Input: part model. Units: mm. Frame: model coordinates. Face numbers are marked on the shaded views. A direction names the side the tool comes from. Coordinates: 2 decimals unless noted, no trailing zeros. Write each loop counter-clockwise with the first axis right and the second up, starting at its lowest first coordinate (ties: lowest second). Pieces come first, ordered by that corner, then holes. Notation, with made-up numbers: (30, -36) - (71, -36) arc R23 ccw to (71, -11) - close; hole circle Ø4 at (14, 64.25). An arc over 180 degrees is marked (long way). Use CSV: the item, a comma, the result in double quotes.
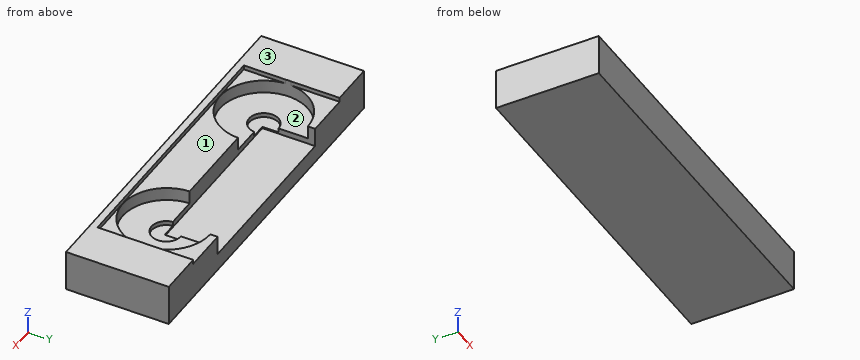
```python
from build123d import *

# Parameters (mm, degrees)
F0_W      = 304.8
F0_H      = 88.9
F1_DEPTH  = 35.56
F2_R      = 38.1
F3_DEPTH  = 15.24
F4_R      = 38.1
F5_DEPTH  = 15.24
F6_W      = 152.4
F6_H      = 20.32
F7_DEPTH  = 45.72
F8_W      = 228.6
F8_H      = 82.7938915014
F9_DEPTH  = 3.81
F10_R     = 12.7
F11_DEPTH = 3.81
F12_R     = 12.7
F13_DEPTH = 3.81


# Not quite as in the source:
# - a feature of the source that left no trace in its solid (it failed there, or was rolled back) is left out


with BuildPart() as f1:
    # F0 (on Top) → F1 (new body)
    with BuildSketch(Plane.XY):
        Rectangle(F0_W, F0_H)
    extrude(amount=F1_DEPTH)

    # F2 (on face) → F3 (cut)
    with BuildSketch(Plane.XY.offset(35.56)):
        with Locations((75.4419565201, 0)):
            Circle(F2_R)
    extrude(amount=-F3_DEPTH, mode=Mode.SUBTRACT)

    # F4 (on face) → F5 (cut)
    with BuildSketch(Plane.XY.offset(35.56)):
        with Locations((-76.2725099921, 0)):
            Circle(F4_R)
    extrude(amount=-F5_DEPTH, mode=Mode.SUBTRACT)

    # F6 (on face) → F7 (cut)
    with BuildSketch(Plane(origin=(0, 44.45, 0), x_dir=(-1, 0, 0), z_dir=(0, 1, 0))):
        with Locations((0, 25.4)):
            Rectangle(F6_W, F6_H)
    extrude(amount=-F7_DEPTH, mode=Mode.SUBTRACT)

    # F8 (on face) → F9 (cut)
    with BuildSketch(Plane.XY.offset(35.56)):
        with Locations((0, 3.0530542493)):
            Rectangle(F8_W, F8_H)
    extrude(amount=-F9_DEPTH, mode=Mode.SUBTRACT)

    # F10 (on face) → F11 (cut)
    with BuildSketch(Plane.XY.offset(20.32)):
        with Locations((-76.2, 0)):
            Circle(F10_R)
    extrude(amount=-F11_DEPTH, mode=Mode.SUBTRACT)

    # F12 (on face) → F13 (cut)
    with BuildSketch(Plane.XY.offset(20.32)):
        with Locations((76.2, 0)):
            Circle(F12_R)
    extrude(amount=-F13_DEPTH, mode=Mode.SUBTRACT)


solid = f1.part
```
(1) Pin query (flat end, axial travel): pin 1 Ø23 at (x, y) = (-76.2, 0) entering from -Z; pin 2 Ø10 at (x, y) = (-24.5, 2) entering from +Z; pin 3 Ø8.5 at (x, z) = (-1, 26.5) entering from +Y; pin 4 Ø12.5 at (x, y) = (76, -5) entering from +Z. Return the tip coordinate at first contact, or that it passes through.
Check values:
pin 1,"z = 0"
pin 2,"z = 31.75"
pin 3,"y = -1.27"
pin 4,"z = 16.51"
(2) Cut plane B-B on y = 26. Return loops of the section in (x, z), and give its area (3 significant figures).
Check values:
outline,"(-152.4, 0) - (152.4, 0) - (152.4, 35.56) - (114.3, 35.56) - (114.3, 31.75) - (103.29, 31.75) - (103.29, 20.32) - (76.2, 20.32) - (76.2, 15.24) - (-76.2, 15.24) - (-76.2, 20.32) - (-104.12, 20.32) - (-104.12, 31.75) - (-114.3, 31.75) - (-114.3, 35.56) - (-152.4, 35.56) - close"
area,"6,820 mm^2"
(3) Cut plane A-A on x = 45. Return loops of the section in (y, z).
Check values:
outline,"(-44.45, 0) - (44.45, 0) - (44.45, 15.24) - (-1.27, 15.24) - (-1.27, 20.32) - (-22.91, 20.32) - (-22.91, 31.75) - (-38.34, 31.75) - (-38.34, 35.56) - (-44.45, 35.56) - close"
(4) Cut plane D-D on x = -14. Return loops of the section in (y, z), and give its area (3 significant figures).
Check values:
outline,"(-44.45, 0) - (44.45, 0) - (44.45, 15.24) - (-1.27, 15.24) - (-1.27, 31.75) - (-38.34, 31.75) - (-38.34, 35.56) - (-44.45, 35.56) - close"
area,"2,090 mm^2"
(5) Cut plane C-C on z = 24. Return loops of the section in (x, y).
Check values:
outline,"(-152.4, -44.45) - (152.4, -44.45) - (152.4, 44.45) - (76.2, 44.45) - (76.2, 38.09) arc R38.1 cw (long way) to (37.36, -1.27) - (-38.19, -1.27) arc R38.1 cw (long way) to (-76.2, 38.1) - (-76.2, 44.45) - (-152.4, 44.45) - close"
(6) Reachability of the marked faces 1, 2 and 3 from +Z, -Z, +X, -X, +Y, -Y: full face, straight path, thin tool, end or side. Return the list, or none.
Check values:
face 1,"+Z, +Y"
face 2,"+Z"
face 3,"+Z, +X, -X, +Y, -Y"
(7) Ray query, probe 1 along X at (y, z) = (0, 19.1); probe 2 along X at (y, z) = (0, 26); probe 3 along Y at (x, z) = (25, 31). Return the intervals inside material, ascending. Write a range as from..to.
Check values:
probe 1,"-152.4..-88.9, 88.9..152.4"
probe 2,"-152.4..-114.37, 113.54..152.4"
probe 3,"-44.45..-1.27"
